Can you work these out from the drawing? Everything is in mm from the part's minimum corner. A direction names the side the tool comes from. Round coordinates to 2 decimals unless told otherwise and drop trailing zeros. Order: outer loops, then holes, each group sorted by start corner. A loop starts at its lowest first (then second) coordinate and runs counter-clockwise, first axis right, second up. Notation, with made-up numbers: (70, -23) -> (87, -23) arc R27 ccw to (87, -6) -> close; hole circle Ø4 at (-17, 40). An arc over 180 degrees is marked (long way). One line per item, written item: value.
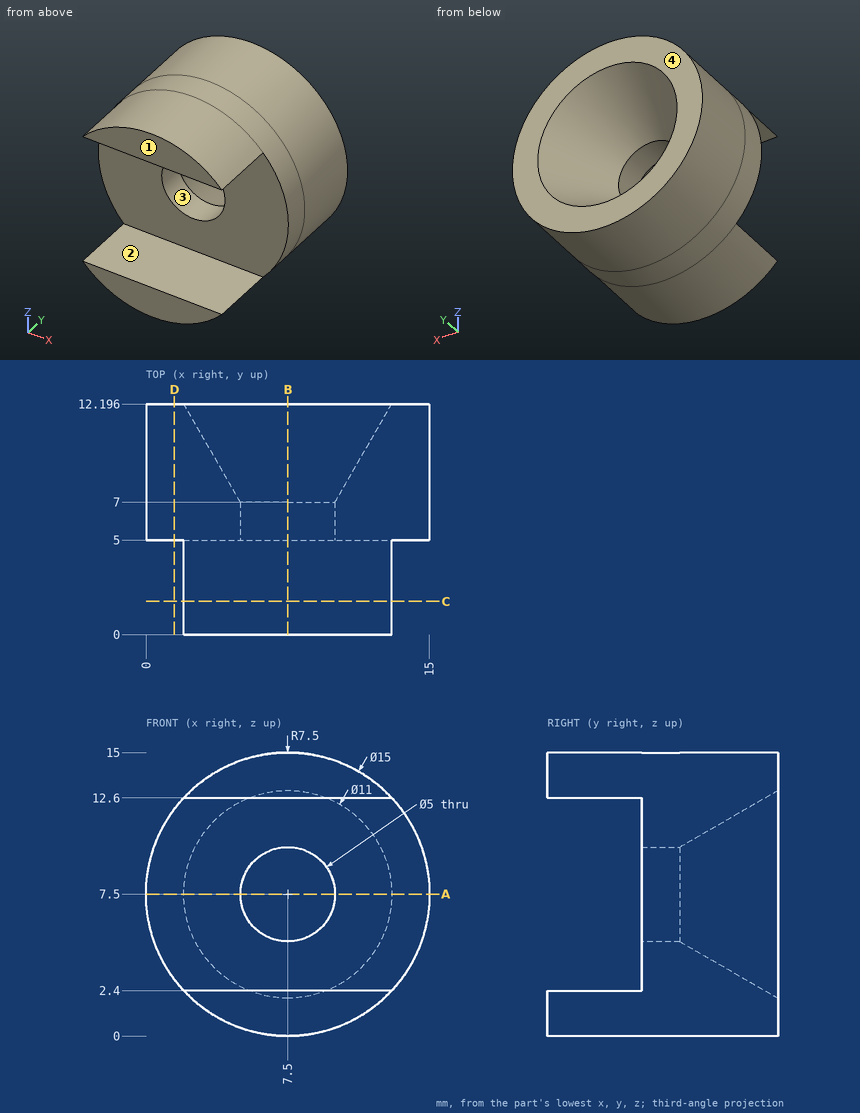
Q1. Which directions (+Z, -Z, +X, -X, +Y, -Y) give clear straight access to the entire face, cutting with the end or side of a thin tool? Please do the marked faces 1 and 2.
Answers:
face 1: +Z, -Z, +X, -X, -Y
face 2: +X, -X, -Y
Q2. I want a section at B-B on x = 7.5. Write out the boundary of the cut face in (y, z).
Answers:
outline: (0, 0) -> (12.2, 0) -> (12.2, 2) -> (7, 5) -> (5, 5) -> (5, 2.4) -> (0, 2.4) -> close; (0, 12.6) -> (5, 12.6) -> (5, 10) -> (7, 10) -> (12.2, 13) -> (12.2, 15) -> (0, 15) -> close
Q3. I want a section at D-D on x = 1.5. Write out the boundary of the cut face in (y, z).
Answers:
outline: (5, 3) -> (12.2, 3) -> (12.2, 12) -> (5, 12) -> close
Q4. I need wall thicknesses on line 1 along Z through (x, y) = (7.5, 6.3); line 2 along Z through (x, y) = (9, 7.25). Which ranges of each line are inside material? Lowest first, please.
Answers:
line 1: 0 to 5, 10 to 15
line 2: 0.15 to 5.32, 9.68 to 14.85
Q5. I want a section at A-A on z = 7.5. Write out the boundary of the cut face in (x, y), then the cut area to 3 significant figures.
Answers:
outline: (0, 5) -> (5, 5) -> (5, 7) -> (2, 12.2) -> (0, 12.2) -> close; (10, 5) -> (15, 5) -> (15, 12.2) -> (13, 12.2) -> (10, 7) -> close
area: 56.4 mm2
Q6. If we mould it in two halves opening along X, with no side actions, what happens to the marked faces 3 and 4? For each: pulls with the +X half, pulls with the -X half, needs draft (parallel to the pull), parting line crosses it, or undercut.
Answers:
face 3: undercut
face 4: needs draft
Q7. For P1, Ø1.5, axis at x = 10, y = 3.5, coming from the -Z side, with a flat end and sliding along its axis, tell me the tip position at first contact or that it passes through.
Answers:
P1: z = 0.21
Q8. I want a section at C-C on y = 1.75. Write out the boundary of the cut face in (x, z).
Answers:
outline: (2, 2.4) arc R7.5 ccw to (13, 2.4) -> close; (2, 12.6) -> (13, 12.6) arc R7.5 ccw to start
